from build123d import *

# Parameters (mm, degrees)
SKETCH1_W               = 42.2
SKETCH1_H               = 15.8
BOSS_EXTRUDE1_DEPTH     = 9.666666667
CUT_EXTRUDE1_DEPTH      = 47.086054772
CUT_EXTRUDE1_DEPTH_BACK = 47.086054772
SKETCH2_R               = 1.125
SKETCH3_W               = 40.1894
SKETCH3_H               = 12.2936
CUT_EXTRUDE3_DEPTH      = 7.745557598
FILLET1_R               = 1.27
CUT_EXTRUDE4_DEPTH      = 46.721698049
CUT_EXTRUDE4_DEPTH_BACK = 46.721698049
SKETCH4_R               = 1.143


with BuildPart() as part:
    # Sketch1 → Boss-Extrude1 (new body)
    with BuildSketch(Plane.XY):
        with Locations((21.1, 7.9)):
            Rectangle(SKETCH1_W, SKETCH1_H)
    extrude(amount=BOSS_EXTRUDE1_DEPTH)

    # Sketch2 → Cut-Extrude1 (cut, two sides: drawn at the far end of the back side and taken through both)
    with BuildSketch(Plane(origin=(42.2, 0, 0), x_dir=(0, 0, -1), z_dir=(1, 0, 0)).offset(-CUT_EXTRUDE1_DEPTH_BACK)):
        with Locations((-5, 12.3)):
            Circle(SKETCH2_R)
    extrude(amount=CUT_EXTRUDE1_DEPTH + CUT_EXTRUDE1_DEPTH_BACK, mode=Mode.SUBTRACT)

    # Sketch3 → Cut-Extrude3 (cut)
    with BuildSketch(Plane.XY.offset(9.666666667)):
        with Locations((21.0947, 6.1468)):
            Rectangle(SKETCH3_W, SKETCH3_H)
    extrude(amount=-CUT_EXTRUDE3_DEPTH, mode=Mode.SUBTRACT)

    # Fillet1
    # the kernel refuses this fillet: 1.27 mm, written as the material it takes off along each edge
    with BuildSketch(Plane(origin=(0, 12.3, 5), x_dir=(0, 0, -1), z_dir=(0, -1, 0))) as fillet1_piece_1:
        with BuildLine():
            CenterArc((1.125 + FILLET1_R, FILLET1_R), FILLET1_R, 180, 90)
            Line((1.125, FILLET1_R), (1.125, 0))
            Line((1.125, 0), (1.125 + FILLET1_R, 0))
        make_face()
    revolve(axis=Axis((0, 12.3, 5), (1, 0, 0)), mode=Mode.SUBTRACT)
    with BuildSketch(Plane(origin=(42.2, 12.3, 5), x_dir=(0, 0, -1), z_dir=(0, -1, 0))) as fillet1_piece_2:
        with BuildLine():
            CenterArc((1.125 + FILLET1_R, -FILLET1_R), FILLET1_R, 90, 90)
            Line((1.125, -FILLET1_R), (1.125, 0))
            Line((1.125, 0), (1.125 + FILLET1_R, 0))
        make_face()
    revolve(axis=Axis((42.2, 12.3, 5), (1, 0, 0)), mode=Mode.SUBTRACT)

    # Sketch4 → Cut-Extrude4 (cut, two sides: drawn at the far end of the back side and taken through both)
    with BuildSketch(Plane.XY.offset(1.921109069).offset(-CUT_EXTRUDE4_DEPTH_BACK)):
        with Locations((6.25, 3.1)):
            Circle(SKETCH4_R)
        with Locations((15.75, 3.1)):
            Circle(SKETCH4_R)
        with Locations((26.45, 3.1)):
            Circle(SKETCH4_R)
        with Locations((35.95, 3.1)):
            Circle(SKETCH4_R)
    extrude(amount=CUT_EXTRUDE4_DEPTH + CUT_EXTRUDE4_DEPTH_BACK, mode=Mode.SUBTRACT)


solid = part.part
For this review, take the finished solid that the model builds, in its own axes (mm). A direction names the side the tool comes from. Give positions to 0.01 mm unless a question says otherwise; leave off trailing zeros. Loops run counter-clockwise (first coordinate to the right, second up) from the corner with the lowest first, then second, coordinate; pieces in that order, holes last. Notation, with made-up numbers: (-26, 43) - (21, 43) arc R12 ccw to (21, 52) - close; hole circle Ø4 at (46, -30). An arc over 180 degrees is marked (long way). Write each question's results on one line, items separated by ' | '.
(1) Take a section at D-D (x = 31). Give the boundary of the cut face in (y, z) (3 decimals), then the cut area to 3 significant figures.
Conclusion:
outline: (0, 0) - (15.8, 0) - (15.8, 9.667) - (12.294, 9.667) - (12.294, 6.125) arc R1.125 cw (long way) to (12.294, 3.875) - (12.294, 1.921) - (0, 1.921) - close | area: 55.5 mm^2
(2) Take a section at B-B (z = 5). Give the boundary of the cut face in (x, y) (3 decimals), then the cut area to 3 significant figures.
Conclusion:
outline: (0, 0) - (1, 0) - (1, 11.146) arc R1.27 ccw to (0, 9.905) - close; (0, 14.695) arc R1.27 ccw to (1.27, 13.425) - (40.93, 13.425) arc R1.27 ccw to (42.2, 14.695) - (42.2, 15.8) - (0, 15.8) - close; (41.189, 0) - (42.2, 0) - (42.2, 9.905) arc R1.27 ccw to (41.189, 11.148) - close | area: 121 mm^2
(3) For pin 1 Ø4 at (x, z) = (7.5, 7) entering from -Y; pin 2 Ø2 at (x, y) = (35.95, 3.1) entering from +Z; pin 3 Ø3 at (x, y) = (6.25, 3.1) entering from +Z, all flat-tipped, find the tip position at first contact; note any pin that passes through.
Conclusion:
pin 1: y = 12.29 | pin 2: through | pin 3: z = 1.92
(4) For faces 1 (the flat face through (21, 6, 1.921)), 2 (the cylindrical face through (27.54, 3.44, 0.95)), list the 3-axis set-ups (+Z, -Z, +X, -X, +Y, -Y) from which the entire face can be reached by the end or side of a thin tool; tool diameter is ignored.
Conclusion:
face 1: +Z, -Y | face 2: +Z, -Z
(5) Take a section at C-C (y = 3.1). Give the boundary of the cut face in (x, z).
Conclusion:
outline: (0, 0) - (5.11, 0) - (5.11, 1.92) - (1, 1.92) - (1, 9.67) - (0, 9.67) - close; (7.39, 0) - (14.61, 0) - (14.61, 1.92) - (7.39, 1.92) - close; (16.89, 0) - (25.31, 0) - (25.31, 1.92) - (16.89, 1.92) - close; (27.59, 0) - (34.81, 0) - (34.81, 1.92) - (27.59, 1.92) - close; (37.09, 0) - (42.2, 0) - (42.2, 9.67) - (41.19, 9.67) - (41.19, 1.92) - (37.09, 1.92) - close
(6) For line 1 along X through (y, z) = (3.1, 1.5); line 2 along X through (y, z) = (9.75, 7.75); line 3 along Y through (x, z) = (26.45, 1.4), list the stretches that pass through material, from the lowest coordinate up.
Conclusion:
line 1: 0 to 5.11, 7.39 to 14.61, 16.89 to 25.31, 27.59 to 34.81, 37.09 to 42.2 | line 2: 0 to 1, 41.19 to 42.2 | line 3: 0 to 1.96, 4.24 to 15.8
(7) Take a section at A-A (x = 26.45). Give the boundary of the cut face in (y, z) (3 decimals), then the cut area to 3 significant figures.
Conclusion:
outline: (0, 0) - (1.957, 0) - (1.957, 1.921) - (0, 1.921) - close; (4.243, 0) - (15.8, 0) - (15.8, 9.667) - (12.294, 9.667) - (12.294, 6.125) arc R1.125 cw (long way) to (12.294, 3.875) - (12.294, 1.921) - (4.243, 1.921) - close | area: 51.1 mm^2
(8) Draft analysis for pull direction Z (two halves, no side actions). For faces 3 (the flat face through (21, 13, 9.667)), 4 (the cylindrical face through (20.822, 13.425, 4.975)), 5 (the flat face through (21, 0, 1)), state which applies: +Z half, -Z half, draft (parallel to the pull), parting line (faces both ways), or undercut.
Conclusion:
face 3: +Z half | face 4: undercut | face 5: draft
